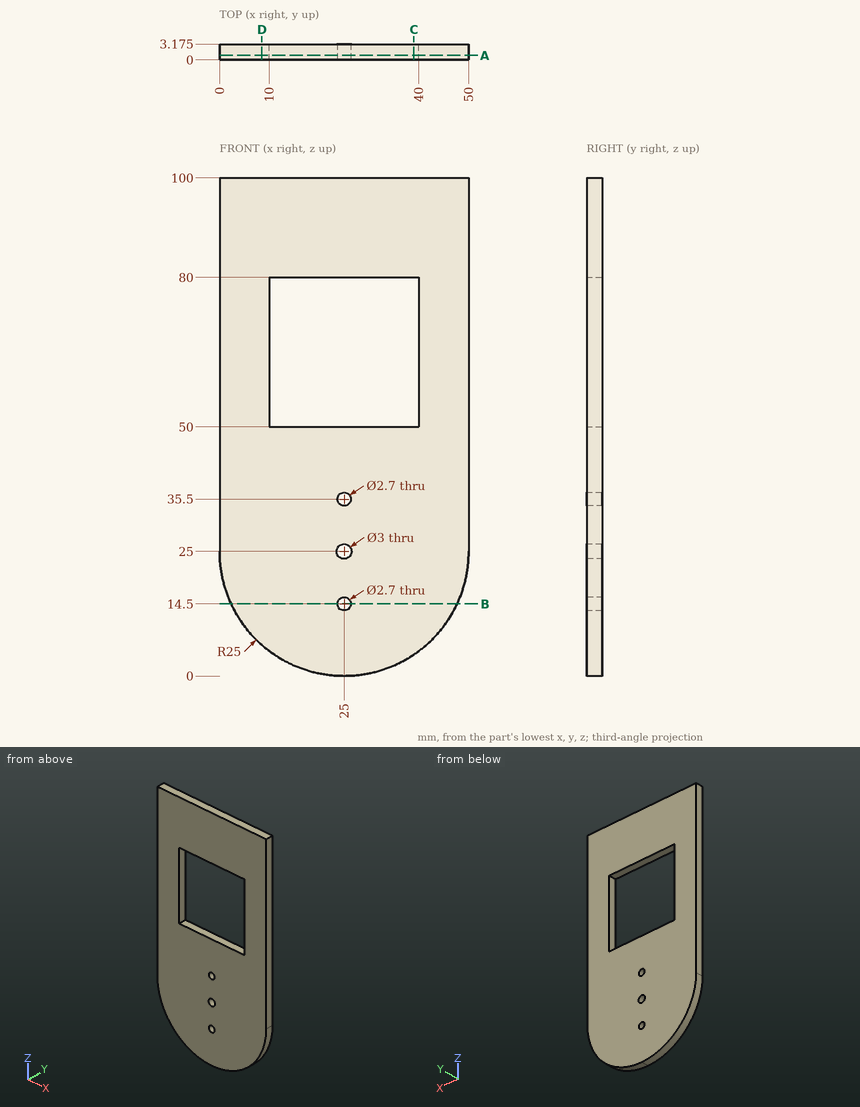
Input: dimensioned drawing with shaded views. Units: mm. Origin: part minimum x, y, z. Coordinates: 2 decimals unless noted, no trailing zeros. Loops run counter-clockwise (first coordinate to the right, second up) from the corner with the lowest first, then second, coordinate; pieces in that order, holes last. Notation, with made-up numbers: M 8.25,64.25 L 40.25,64.25 A21 cw 40.25,77.25 Z; hole C -23.5,55.5 d8. An arc over 180 degrees is marked long. One line per item, written item: value. Start each with the question number.
1) Material intervals for L1, parallel to X at y = 1.2, z = 25; L2, parallel to X at y = 2.2, z = 35.5; L3, parallel to Z at x = 30, y = 1, sorted ascending. Write a range as from..to.
2) Cut plane C-C (x = 39). Return loops of the section in (y, z) (3 decimals).
3) Pin query (flat end, axial travel): P1, Ø1.6, axis at x = 25, z = 14.5, coming from the +Y side; P2, Ø1, axis at x = 28, y = 1.5, coming from the -Z side; P3, Ø1.5, axis at x = 13, y = 2, coming from the -Z side. Return the tip coordinate at first contact, or that it passes through.
4) Cut plane B-B (z = 14.5). Return loops of the section in (x, y) (3 decimals).
5) Cut plane D-D (x = 8.5). Return loops of the section in (y, z) (3 decimals).
6) Cut plane A-A (y = 0.9). Return loops of the section in (x, z), then the cut area to 3 significant figures.
Evaluation:
1. L1: 0..23.5, 26.5..50
1. L2: 0..23.65, 26.35..50
1. L3: 0.51..50, 80..100
2. outline: M 0,4.288 L 3.175,4.288 L 3.175,50 L 0,50 Z; M 0,80 L 3.175,80 L 3.175,100 L 0,100 Z
3. P1: through
3. P2: z = 0.13
3. P3: z = 2.67
4. outline: M 2.312,0 L 23.65,0 L 23.65,3.175 L 2.312,3.175 Z; M 26.35,0 L 47.688,0 L 47.688,3.175 L 26.35,3.175 Z
5. outline: M 0,6.218 L 3.175,6.218 L 3.175,100 L 0,100 Z
6. outline: M 0,25 A25 ccw 50,25 L 50,100 L 0,100 Z; hole M 10,50 L 40,50 L 40,80 L 10,80 Z; hole C 25,25 d3; hole C 25,14.5 d2.7; hole C 25,35.5 d2.7
6. area: 3,810 mm^2
